from build123d import *

# Parameters (mm, degrees)
BOSS_EXTRUDE1_DEPTH = 6
SKETCH2_R           = 9
BOSS_EXTRUDE2_DEPTH = 1
SKETCH3_R           = 5
BOSS_EXTRUDE3_DEPTH = 45


with BuildPart() as part:
    # Sketch1 → Boss-Extrude1 (new body)
    with BuildSketch(Plane.XY):
        Polygon((0, 9), (-7.794228634, 4.5), (-7.794228634, -4.5), (0, -9), (7.794228634, -4.5), (7.794228634, 4.5), align=None)
    extrude(amount=BOSS_EXTRUDE1_DEPTH)

    # Sketch2 → Boss-Extrude2 (add)
    with BuildSketch(Plane(origin=(0, 0, 0), x_dir=(-1, 0, 0), z_dir=(0, 0, -1))):
        Circle(SKETCH2_R)
    extrude(amount=BOSS_EXTRUDE2_DEPTH)

    # Sketch3 → Boss-Extrude3 (add)
    with BuildSketch(Plane(origin=(0, 0, -1), x_dir=(-1, 0, 0), z_dir=(0, 0, -1))):
        Circle(SKETCH3_R)
    extrude(amount=BOSS_EXTRUDE3_DEPTH)


solid = part.part
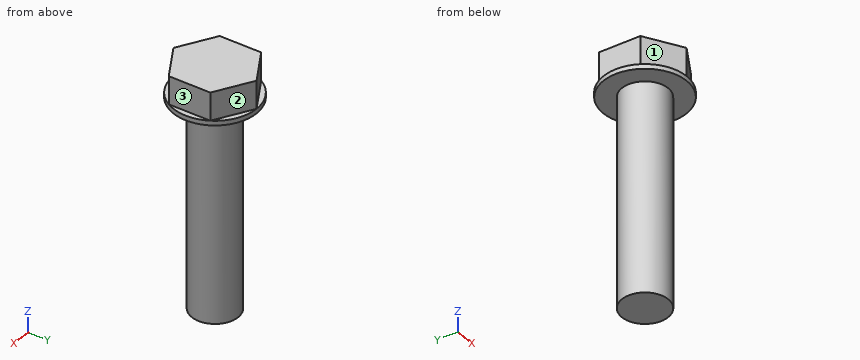
Work out the finished part from the listing and answer in its coordinate system (mm). Face numbers are marked on the shaded views. A direction names the side the tool comes from. Coordinates: 2 decimals unless noted, no trailing zeros. Write each loop counter-clockwise with the first axis right and the second up, starting at its lowest first coordinate (ties: lowest second). Pieces come first, ordered by that corner, then holes.
1. The part is cut by section A-A, the plane y = 0. Write down the section's boundary in (x, z), and give its area (3 significant figures).
Results list:
outline: (-9, -1) - (-5, -1) - (-5, -46) - (5, -46) - (5, -1) - (9, -1) - (9, 0) - (7.79, 0) - (7.79, 6) - (-7.79, 6) - (-7.79, 0) - (-9, 0) - close
area: 562 mm2
2. The part is cut by section D-D, the plane y = -6.25. Write down the section's boundary in (x, z).
Results list:
outline: (-6.48, -1) - (6.48, -1) - (6.48, 0) - (4.76, 0) - (4.76, 6) - (-4.76, 6) - (-4.76, 0) - (-6.48, 0) - close
3. The part is cut by section C-C, the plane z = -32. Write down the section's boundary in (x, y).
Results list:
outline: circle Ø10 at (0, 0)
4. Consider line 1 along Z through (x, y) = (2.75, 6.25); line 2 along Y through (x, z) = (0.25, -32.5); line 3 along Y through (x, z) = (5.5, 1). Determine where each line is inside the solid, lowest interval first.
Results list:
line 1: z = -1 to 6
line 2: y = -4.99 to 4.99
line 3: y = -5.82 to 5.82
5. For the marked faces 1, 2 and 3, determine the directions among +Z, -Z, +X, -X, +Y, -Y from which every point of the face is accessible in a straight line to the end or side of a thin tool.
Results list:
face 1: +Z, -X, -Y
face 2: +Z, +X, +Y
face 3: +Z, +X, +Y, -Y
6. Flat-ended cylindrical pins translate along their axes: pin 1 (2 mm diameter, centred on y = -5.5, z = -12, fed in from -X); pin 2 (6.5 mm diameter, centred on y = 1.5, z = 4.5, fed in from +X); pin 3 (6 mm diameter, centred on x = -0.5, z = -39.5, fed in from -Y). Find the tip coordinate at first contact, or state that the pin passes through.
Results list:
pin 1: stops at x = -2.18
pin 2: stops at x = 7.79
pin 3: stops at y = -5
7. The part is cut by section B-B, the plane x = 5.5. Write down the section's boundary in (y, z).
Results list:
outline: (-7.12, -1) - (7.12, -1) - (7.12, 0) - (5.82, 0) - (5.82, 6) - (-5.82, 6) - (-5.82, 0) - (-7.12, 0) - close
